Part print with two shaded views. Sizes in mm from the minimum x, y, z corner. A direction names the side the tool comes from. Round coordinates to 2 decimals unless told otherwise and drop trailing zeros. Order: outer loops, then holes, each group sorted by start corner. A loop starts at its lowest first (then second) coordinate and runs counter-clockwise, first axis right, second up. Notation, with made-up numbers: (-40, 1) -> (-14, 1) arc R16 ccw to (-14, 18) -> close; hole circle Ø6 at (-25, 42). An arc over 180 degrees is marked (long way). Use a Markdown table: item, result. Add a question column.
Item 1: Slice it at A-A, the plane y = 2.75. Give the cut face in (x, z).
Item 2: 3-axis set-ups, long thin cutter, end or side, ignore diameter. For the marked faces 4 and 5: which of +Z, -Z, +X, -X, +Y, -Y reach the whole face in a straight line?
Item 3: Two-plate mould, pull along Y, no slides. Class the marked faces 1, 2 and 3: released by +Y, released by -Y, zero draft, split by the parting line, or undercut.
Item 4: Pin check, flat tip, straight feed: pin 1 (2 mm diameter, centred on x = 2, z = 2.5, fed in from -Y). Stop position of the tip, or through.
Item 5: Probe L1, parallel to Z at x = 3.4, y = 0.75; L2, parallel to Y at x = 2.75, z = 2; L3, parallel to Z at x = 2, y = 3.55. List the from-to ranges inside material, lowest first.
Item 6: Slice it at B-B, the plane z = 1.5. Give the cut face in (x, y).
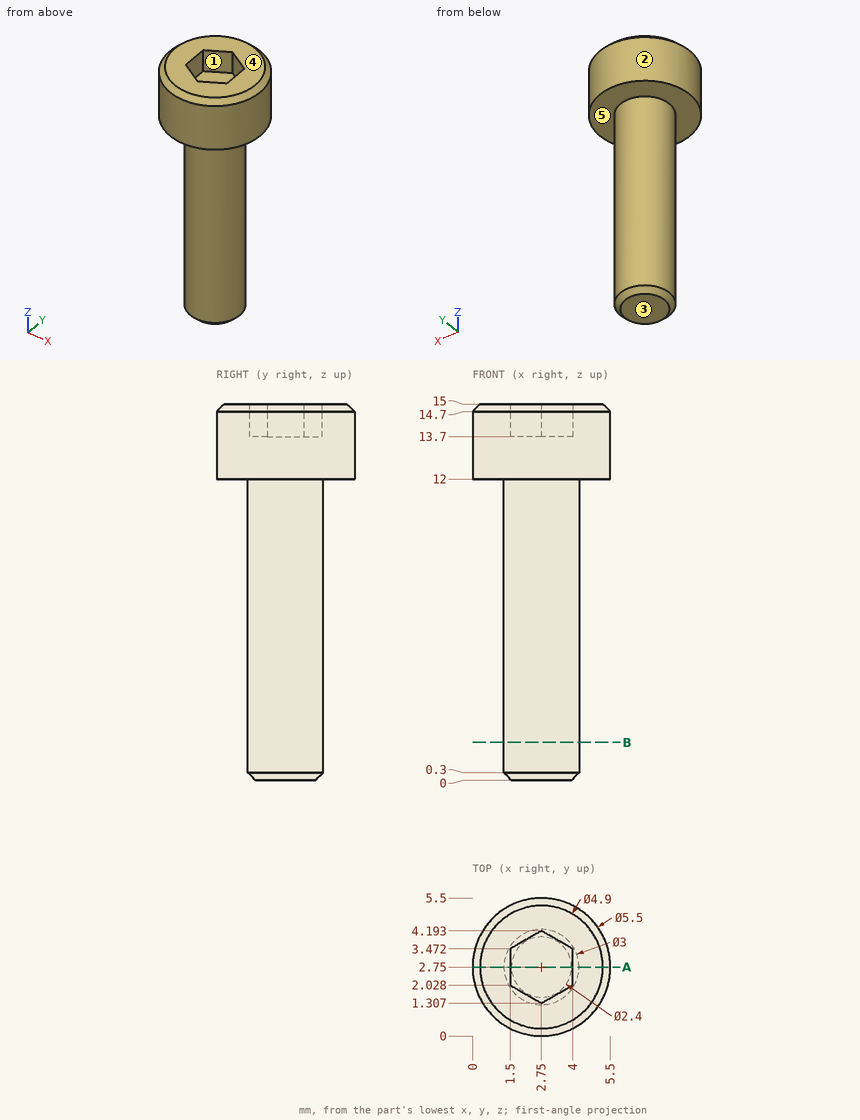
Check sheet entries:
| question | item | result |
|---|---|---|
| 1 | outline | (0, 12) -> (1.25, 12) -> (1.25, 0.3) -> (1.55, 0) -> (3.95, 0) -> (4.25, 0.3) -> (4.25, 12) -> (5.5, 12) -> (5.5, 14.7) -> (5.2, 15) -> (4, 15) -> (4, 13.7) -> (1.5, 13.7) -> (1.5, 15) -> (0.3, 15) -> (0, 14.7) -> close |
| 2 | face 4 | +Z, +X, -X, +Y, -Y |
| 2 | face 5 | -Z |
| 3 | face 1 | undercut |
| 3 | face 2 | split by the parting line |
| 3 | face 3 | zero draft |
| 4 | pin 1 | y = 1.25 |
| 5 | L1 | 12 to 15 |
| 5 | L2 | 1.25 to 4.25 |
| 5 | L3 | 0 to 13.7 |
| 6 | outline | circle Ø3 at (2.75, 2.75) |
